Geometry: final body of the model. Coordinates: model frame, mm. Face numbers are marked on the shaded views. Give positions to 0.01 mm unless a question says otherwise; leave off trailing zeros. Order: outer loops, then holes, each group sorted by start corner. A loop starts at its lowest first (then second) coordinate and runs counter-clockwise, first axis right, second up. Notation, with made-up numbers: (42, 89) - (67, 89) arc R24 ccw to (67, 112) - close; hole circle Ø7 at (-24.75, -35.75). An arc over 180 degrees is marked (long way). One line per item, written item: value.
```python
from build123d import *

# Parameters (mm, degrees)
SKETCH1_W               = 46.355
SKETCH1_H               = 46.355
BOSS_EXTRUDE1_DEPTH     = 63.5
SKETCH2_R               = 1.27
CUT_EXTRUDE1_DEPTH      = 64.5
SKETCH4_R               = 3.4925
CUT_EXTRUDE3_DEPTH      = 64.5
MIRROR2_COPY_1_SKETCH_R = 3.4925
MIRROR2_COPY_1_DEPTH    = 64.5
SKETCH6_W               = 50.639915967
SKETCH6_H               = 51.332427637
CUT_EXTRUDE4_DEPTH      = 25.4


with BuildPart() as part:
    # Sketch1 → Boss-Extrude1 (new body)
    with BuildSketch(Plane.XY):
        Rectangle(SKETCH1_W, SKETCH1_H)
    extrude(amount=BOSS_EXTRUDE1_DEPTH)

    # Sketch2 → Cut-Extrude1 (cut, through all)
    with BuildSketch(Plane.XY.offset(63.5)):
        Circle(SKETCH2_R)
    extrude(amount=-CUT_EXTRUDE1_DEPTH, mode=Mode.SUBTRACT)

    # Sketch4 → Cut-Extrude3 (cut, through all)
    with BuildSketch(Plane.XY.offset(63.5)):
        with Locations((14.601896453, 14.601896453)):
            Circle(SKETCH4_R)
    cut_extrude3 = extrude(amount=-CUT_EXTRUDE3_DEPTH, mode=Mode.SUBTRACT)

    # Mirror1: Cut-Extrude3 across plane
    add(cut_extrude3.mirror(Plane.ZX), mode=Mode.SUBTRACT)

    # Mirror2: Cut-Extrude3 across plane
    add(cut_extrude3.mirror(Plane(origin=(0, 0, 0), x_dir=(0, 0, 1), z_dir=(1, 0, 0))), mode=Mode.SUBTRACT)

    # Mirror2 copy 1 sketch → Mirror2 copy 1 (cut, through all)
    with BuildSketch(Plane(origin=(0, 0, 63.5), x_dir=(-1, 0, 0), z_dir=(0, 0, 1))):
        with Locations((14.601896453, 14.601896453)):
            Circle(MIRROR2_COPY_1_SKETCH_R)
    extrude(amount=-MIRROR2_COPY_1_DEPTH, mode=Mode.SUBTRACT)

    # Sketch5 → Cut-Revolve1 (revolve, cut)
    with BuildSketch(Plane(origin=(0, 0, 0), x_dir=(0, 0, -1), z_dir=(1, 0, 0))):
        Polygon((-63.5, 9.713622118), (-44.057941111, 9.713622118), (0, 1.27), (0, 0), (-63.5, 0), align=None)
    revolve(axis=Axis((0, 0, 0), (0, 0, 1)), mode=Mode.SUBTRACT)

    # Sketch6 → Cut-Extrude4 (cut)
    with BuildSketch(Plane.XY.offset(63.5)):
        with Locations((0.281332866, -0.281332866)):
            Rectangle(SKETCH6_W, SKETCH6_H)
    extrude(amount=-CUT_EXTRUDE4_DEPTH, mode=Mode.SUBTRACT)


solid = part.part
```
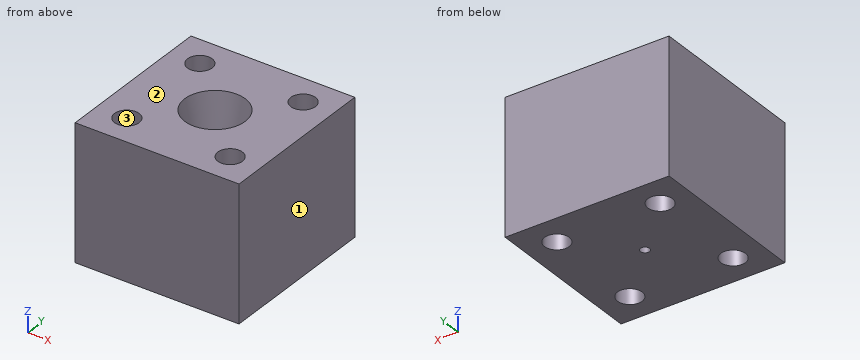
1) Section C-C, the plane z = 14.5. Return loops of the section in (x, y) (1 decimal), then the cut area to 3 significant figures.
Answers below:
outline: (-23.2, -23.2) - (23.2, -23.2) - (23.2, 23.2) - (-23.2, 23.2) - close; hole circle Ø7 at (-14.6, -14.6); hole circle Ø7 at (-14.6, 14.6); hole circle Ø8.1 at (0, 0); hole circle Ø7 at (14.6, -14.6); hole circle Ø7 at (14.6, 14.6)
area: 1,940 mm^2
2) Section A-A, the plane y = 0. Return loops of the section in (x, z), then the cut area to 3 significant figures.
Answers below:
outline: (-23.18, 0) - (-1.27, 0) - (-8.57, 38.1) - (-23.18, 38.1) - close; (1.27, 0) - (23.18, 0) - (23.18, 38.1) - (8.57, 38.1) - close
area: 1,390 mm^2
3) Section D-D, the plane x = -15. Return loops of the section in (y, z).
Answers below:
outline: (-23.18, 0) - (-18.07, 0) - (-18.07, 38.1) - (-23.18, 38.1) - close; (-11.13, 0) - (11.13, 0) - (11.13, 38.1) - (-11.13, 38.1) - close; (18.07, 0) - (23.18, 0) - (23.18, 38.1) - (18.07, 38.1) - close
4) Material intervals for line 1 along Y through (x, z) = (-14.5, 9); line 2 along Y through (x, z) = (12.5, 10.5); line 3 along X through (y, z) = (0, 36), sorted ascending.
Answers below:
line 1: -23.18 to -18.09, -11.11 to 11.11, 18.09 to 23.18
line 2: -23.18 to -17.39, -11.81 to 11.81, 17.39 to 23.18
line 3: -23.18 to -8.17, 8.17 to 23.18
5) Mould query, pull axis X, two halves, no side actions, for the marked faces 1, 2 and 3. Classes: released by +X, released by -X, zero draft, split by the parting line, or undercut.
Answers below:
face 1: released by +X
face 2: zero draft
face 3: undercut
